```python
from build123d import *

# Parameters (mm, degrees)
ESBO_O1_W                = 6
ESBO_O1_H                = 10
RESSALTO_EXTRUS_O1_DEPTH = 67
ESBO_O2_R                = 2.5
CORTE_EXTRUS_O1_DEPTH    = 67
ESBO_O3_R                = 2
CORTE_EXTRUS_O2_DEPTH    = 6


with BuildPart() as part:
    # Esboço1 → Ressalto-extrusão1 (new body)
    with BuildSketch(Plane.XY):
        with Locations((-3, 5)):
            Rectangle(ESBO_O1_W, ESBO_O1_H)
    extrude(amount=RESSALTO_EXTRUS_O1_DEPTH)

    # Esboço2 → Corte-extrusão1 (cut)
    with BuildSketch(Plane(origin=(0, 0, 0), x_dir=(0, 0, -1), z_dir=(1, 0, 0))):
        with Locations((-63.5, 4.977459114)):
            Circle(ESBO_O2_R)
        with Locations((-56.85, 4.977459114)):
            Circle(ESBO_O2_R)
        with Locations((-50.2, 4.977459114)):
            Circle(ESBO_O2_R)
        with Locations((-43.55, 4.977459114)):
            Circle(ESBO_O2_R)
        with Locations((-36.9, 4.977459114)):
            Circle(ESBO_O2_R)
        with Locations((-30.25, 4.977459114)):
            Circle(ESBO_O2_R)
        with Locations((-23.6, 4.977459114)):
            Circle(ESBO_O2_R)
        with Locations((-16.95, 4.977459114)):
            Circle(ESBO_O2_R)
        with Locations((-10.3, 4.977459114)):
            Circle(ESBO_O2_R)
        with Locations((-3.65, 4.977459114)):
            Circle(ESBO_O2_R)
    extrude(amount=-CORTE_EXTRUS_O1_DEPTH, mode=Mode.SUBTRACT)

    # Esboço3 → Corte-extrusão2 (cut)
    with BuildSketch(Plane(origin=(0, 10, 0), x_dir=(1, 0, 0), z_dir=(0, 1, 0))):
        with Locations((-3, -63.5)):
            Circle(ESBO_O3_R)
        with Locations((-3, -56.85)):
            Circle(ESBO_O3_R)
        with Locations((-3, -50.2)):
            Circle(ESBO_O3_R)
        with Locations((-3, -43.55)):
            Circle(ESBO_O3_R)
        with Locations((-3, -36.9)):
            Circle(ESBO_O3_R)
        with Locations((-3, -30.25)):
            Circle(ESBO_O3_R)
        with Locations((-3, -23.6)):
            Circle(ESBO_O3_R)
        with Locations((-3, -16.95)):
            Circle(ESBO_O3_R)
        with Locations((-3, -10.3)):
            Circle(ESBO_O3_R)
        with Locations((-3, -3.65)):
            Circle(ESBO_O3_R)
    extrude(amount=-CORTE_EXTRUS_O2_DEPTH, mode=Mode.SUBTRACT)


solid = part.part
```
Could you check a few things on this model? Use its own coordinates, in mm. A direction names the side the tool comes from. Give positions to 0.01 mm unless a question says otherwise; leave off trailing zeros. Loops run counter-clockwise (first coordinate to the right, second up) from the corner with the lowest first, then second, coordinate; pieces in that order, holes last. Notation, with made-up numbers: (-18, 64.25) - (17, 64.25) arc R12 cw to (17, 69.25) - close; hole circle Ø7 at (4.5, -22). An arc over 180 degrees is marked (long way). Use one line per item in the form item = value.
1. I want a section at A-A (z = 63.5). Please give me the cut outline in (x, y).
Response values:
outline = (-6, 0) - (0, 0) - (0, 2.48) - (-6, 2.48) - close; (-6, 7.48) - (-5, 7.48) - (-5, 10) - (-6, 10) - close; (-1, 7.48) - (0, 7.48) - (0, 10) - (-1, 10) - close
2. On a 3-axis mill with a long thin cutter (end or side, diameter ignored), from which of +Z, -Z, +X, -X, +Y, -Y can I reach the whole of each face in a straight line? I mean faces 1 (the face through (-4.474, 8.655, 28.898)), 2 (the face through (-2.958, 2.537, 37.442)). Say none if no direction works.
Response values:
face_1 = +Y
face_2 = +X, -X
3. I'm going to push flat-ended pins straight in: pin 1 Ø4.5 at (y, z) = (4.98, 50.2) entering from -X; pin 2 Ø3.5 at (x, z) = (-3, 50.2) entering from +Y. Where does each tip first touch, or does it pass through?
Response values:
pin_1 = through
pin_2 = 3.19
4. I want a section at B-B (y = 5.75). Give the number of separate pieces and of enclosed holes in the cut face, and give its area (3 significant figures).
Response values:
separate_pieces = 11
enclosed_holes = 0
area = 117 mm²
5. Thinking about a two-plate mould opening in Y: for faces 3 (the face through (-3, 0, 33)), 4 (the face through (-2.958, 2.537, 30.792)), 5 (the face through (-2.958, 2.537, 17.492)), 6 (the face through (-4.474, 8.655, 55.498)), which applies, released by +Y, released by -Y, zero draft, split by the parting line, or undercut?
Response values:
face_3 = released by -Y
face_4 = undercut
face_5 = undercut
face_6 = zero draft
6. I need wall thicknesses on probe 1 along Y at (x, z) = (-0.25, 50); probe 2 along Y at (x, z) = (-3.75, 50.2); probe 3 along X at (y, z) = (8.5, 42). Which ranges of each line are inside material? Lowest first, please.
Response values:
probe_1 = 0 to 2.49, 7.47 to 10
probe_2 = 0 to 2.48
probe_3 = -6 to -4.26, -1.74 to 0
